```python
from build123d import *

# Parameters (mm, degrees)
F0_R     = 4
F0_R_2   = 1.5
F1_DEPTH = 7
F2_R     = 7.4
F3_DEPTH = 3
F4_SIZE  = 1.5
F6_DEPTH = 3


with BuildPart() as f1:
    # F0 (on Top) → F1 (new body)
    with BuildSketch(Plane.XY):
        with BuildLine():
            ThreePointArc((4.0311035144, -4.4441202117), (5.48573701, -2.4303681731), (6, 0))
            ThreePointArc((6, 0), (2.0737198646, 5.6302474122), (-4.5665619744, 3.8918519671))
            ThreePointArc((-4.5665619744, 3.8918519671), (-5.9006846613, 1.0871616841), (-5.6537236585, -2.0088326942))
            ThreePointArc((-5.6537236585, -2.0088326942), (-4.1765759878, -4.3076923077), (-1.8331692436, -5.7130981546))
            ThreePointArc((-1.8331692436, -5.7130981546), (1.2689779429, -5.864272758), (4.0311035144, -4.4441202117))
        make_face()
        Circle(F0_R, mode=Mode.SUBTRACT)
        with BuildLine():
            ThreePointArc((-5.6537236585, -2.0088326942), (-5.9006846613, 1.0871616841), (-4.5665619744, 3.8918519671))
            Line((-4.5665619744, 3.8918519671), (-29.8115717394, -25.7297530192))
            ThreePointArc((-29.8115717394, -25.7297530192), (-27.6751829567, -24.5399699331), (-25.2813289713, -25.0391732176))
            Line((-25.2813289713, -25.0391732176), (-5.6537236585, -2.0088326942))
        make_face()
        with BuildLine():
            Line((-24.7962668709, -30.5924034568), (4.0311035144, -4.4441202117))
            ThreePointArc((4.0311035144, -4.4441202117), (1.2689779429, -5.864272758), (-1.8331692436, -5.7130981546))
            Line((-1.8331692436, -5.7130981546), (-24.2460046276, -26.0429846518))
            ThreePointArc((-24.2460046276, -26.0429846518), (-23.8006490966, -26.9767912058), (-23.647743921, -28))
            ThreePointArc((-23.647743921, -28), (-23.9477306651, -29.4177147676), (-24.7962668709, -30.5924034568))
        make_face()
        with BuildLine():
            ThreePointArc((-25.2813289713, -25.0391732176), (-27.6751829567, -24.5399699331), (-29.8115717394, -25.7297530192))
            ThreePointArc((-29.8115717394, -25.7297530192), (-29.5840799139, -30.5128205128), (-24.7962668709, -30.5924034568))
            ThreePointArc((-24.7962668709, -30.5924034568), (-23.9477306651, -29.4177147676), (-23.647743921, -28))
            ThreePointArc((-23.647743921, -28), (-23.8006490966, -26.9767912058), (-24.2460046276, -26.0429846518))
            ThreePointArc((-24.2460046276, -26.0429846518), (-24.7114079281, -25.4871794872), (-25.2813289713, -25.0391732176))
        make_face()
        with Locations((-27.147743921, -28)):
            Circle(F0_R_2, mode=Mode.SUBTRACT)
    extrude(amount=F1_DEPTH)

    # F2 (on face) → F3 (cut)
    with BuildSketch(Plane.XY.offset(7)):
        with Locations((0, 0.9179179191)):
            Circle(F2_R)
    extrude(amount=-F3_DEPTH, mode=Mode.SUBTRACT)

    # F4
    f4_edges = [f1.edges().sort_by_distance(p)[0] for p in [
        (-28.647744, -28, 7),
    ]]
    chamfer(f4_edges, length=F4_SIZE)

    # F5 (on face) → F6 (cut)
    with BuildSketch(Plane(origin=(-4.5665619744, 3.8918519671, 0), x_dir=(-0.6486419945, -0.7610936624, 0), z_dir=(-0.7610936624, 0.6486419945, 0))):
        Polygon((40.5807819354, 0), (38.9197893108, 7), (38.9197893108, 0), align=None)
        Polygon((38.9197893108, 0), (38.9197893108, 7), (37.0698095831, 7), (38.7308022077, 0), align=None)
    extrude(amount=-F6_DEPTH, mode=Mode.SUBTRACT)


solid = f1.part
```
Geometry check sheet. Reference: the model listing, model coordinates, mm. A direction names the side the tool comes from. Coordinates: 2 decimals unless noted, no trailing zeros. Order: outer loops, then holes, each group sorted by start corner. A loop starts at its lowest first (then second) coordinate and runs counter-clockwise, first axis right, second up. Notation, with made-up numbers: (45, 63.5) - (57, 63.5) arc R31 ccw to (57, 99.5) - close; hole circle Ø5 at (-35.5, -38). An arc over 180 degrees is marked (long way). Answer as a JSON object with one key per item and string values. Group by question number.
Item 1: Tool access check on faces 5 (the face through (-29.61, -27.25, 2.67)), 6 (the face through (-14, -11, 0)), 7 (the face through (-0.11, -6.48, 5.52)). Record the directions out of +Z, -Z, +X, -X, +Y, -Y that give a thin tool (end or side, any length) a straight path to the whole face; none if there is none.
Item 2: Scan lines: probe 1 along X at (y, z) = (0, 1.25); probe 2 along Y at (x, z) = (-13.5, 3.75); probe 3 along Z at (x, y) = (2, -6). Record each from-to range of solid material in increasing order.
Item 3: Draft check along X on faces 1 (the face through (-16.95, -10.64, 3.45)), 2 (the face through (-12.883, -15.736, 3.451)), 3 (the face through (-26.31, -29.55, 5.76)), 4 (the face through (-7.1, -1.17, 5.52)). Enter one of: +X half, -X half, draft (parallel to the pull), parting line (faces both ways), or undercut.
Item 4: Sectioned sample at C-C, the plane z = 6.25. Record the cut outline in (x, y), and give its area (3 significant figures).
Item 5: Sectioned sample at B-B, the plane y = -28. Record the cut outline in (x, z), and give its area (3 significant figures).
Item 6: Sectioned sample at A-A, the plane x = 3. Record the cut outline in (y, z), and give its area (3 significant figures).
Item 7: Depth check by flat-ended pin: pin 1 Ø7 at (x, y) = (0, 0) entering from -Z; pin 2 Ø1 at (x, z) = (2, 3) entering from -Y; pin 3 Ø10 at (x, y) = (-2.5, 2) entering from +Z; pin 4 Ø2 at (y, z) = (-4.5, 2.5) entering from +X. Enter the tip coordinate at first touch or a pass-through.
Item 8: Sectioned sample at D-D, the plane x = -16. Record the cut outline in (y, z), and give its area (3 significant figures).
Resolved:
{
 "1": {"face 5": "-Z", "face 6": "-Z, +X, -X, +Y, -Y", "face 7": "+Z, +Y"},
 "2": {"probe 1": "-7.88 to -4, 4 to 6", "probe 2": "-20.35 to -16.3, -11.22 to -6.59", "probe 3": "0 to 4"},
 "3": {"face 1": "-X half", "face 2": "undercut", "face 3": "undercut", "face 4": "+X half"},
 "4": {"outline": "(-29.92, -25.87) arc R3.5 ccw to (-24.8, -30.59) - (2.13, -6.17) arc R7.4 cw to (-2.28, -6.12) - (-24.25, -26.04) arc R3.5 ccw to (-25.28, -25.04) - (-6.37, -2.85) arc R7.4 cw to (-7.39, 0.58) - (-28.73, -24.46) - (-27.21, -25.75) arc R2.25 cw (long way) to (-28.97, -26.68) - close", "area": "208 mm^2"},
 "5": {"outline": "(-30.65, 0) - (-29.71, 0) - (-28.65, 2.9) - (-28.65, 5.5) - (-30.15, 7) - (-30.65, 7) - close; (-25.65, 0) - (-21.94, 0) - (-21.94, 7) - (-24.15, 7) - (-25.65, 5.5) - close", "area": "36.2 mm^2"},
 "6": {"outline": "(-5.38, 0) - (-2.65, 0) - (-2.65, 4) - (-5.38, 4) - close; (2.65, 0) - (5.2, 0) - (5.2, 4) - (2.65, 4) - close", "area": "21.1 mm^2"},
 "7": {"pin 1": "through", "pin 2": "y = -6.74", "pin 3": "z = 4", "pin 4": "x = 4.87"},
 "8": {"outline": "(-22.61, 0) - (-18.56, 0) - (-18.56, 7) - (-22.61, 7) - close; (-14.15, 0) - (-9.52, 0) - (-9.52, 7) - (-14.15, 7) - close", "area": "60.7 mm^2"}
}
